Check sheet for the drawn part. Datum: minimum x, y, z corner. Units: mm. A direction names the side the tool comes from. Round coordinates to 2 decimals unless told otherwise and drop trailing zeros. Write each loop counter-clockwise with the first axis right and the second up, starting at its lowest first coordinate (ties: lowest second). Pieces come first, ordered by that corner, then holes.
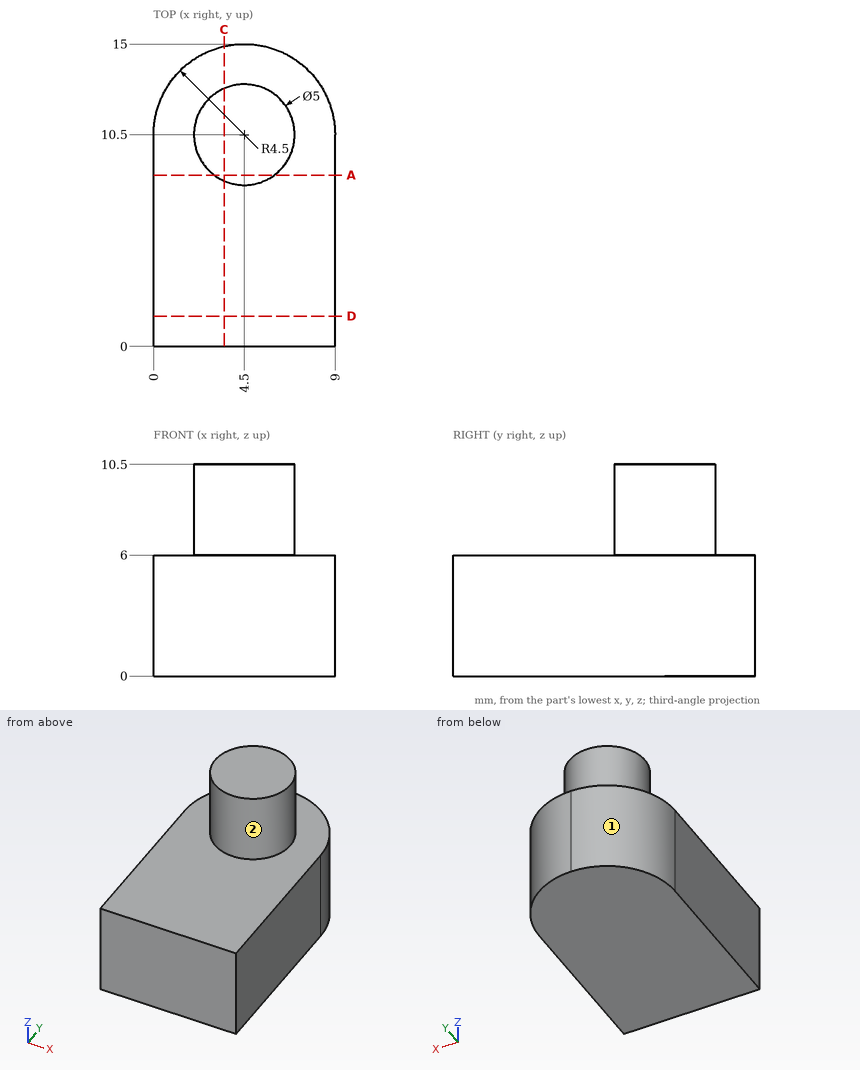
Q1. Tool access check on the marked faces 1 and 2. Record the directions out of +Z, -Z, +X, -X, +Y, -Y that give a thin tool (end or side, any length) a straight path to the whole face; none if there is none.
Recorded:
face 1: +Z, -Z, -X, +Y
face 2: +Z
Q2. Depth check by flat-ended pin: P1, Ø4, axis at x = 2.5, y = 4.5, coming from the -Z side; P2, Ø4, axis at y = 8.5, z = 9, coming from the -X side; P3, Ø1, axis at y = 6, z = 7, coming from the -X side; P4, Ø4, axis at x = 1.5, z = 3.5, coming from the +Y side. Enter the tip coordinate at first touch or a pass-through.
Recorded:
P1: stops at z = 0
P2: stops at x = 2
P3: passes through
P4: stops at y = 14.89
Q3. Material ranges on line 1 along Z through (x, y) = (2, 1.5); line 2 along Y through (x, z) = (4.75, 10); line 3 along X through (y, z) = (14, 4.25), recorded low to high.
Recorded:
line 1: z = 0 to 6
line 2: y = 8.01 to 12.99
line 3: x = 1.67 to 7.33
Q4. Sectioned sample at A-A (y = 8.5). Enter the section's corners in (x, z), plus the area to 3 significant figures.
Recorded:
outline: (0, 0) - (9, 0) - (9, 6) - (6, 6) - (6, 10.5) - (3, 10.5) - (3, 6) - (0, 6) - close
area: 67.5 mm2
Q5. Sectioned sample at C-C (x = 3.5). Enter the section's corners in (y, z), plus the area to 3 significant figures.
Recorded:
outline: (0, 0) - (14.89, 0) - (14.89, 6) - (12.79, 6) - (12.79, 10.5) - (8.21, 10.5) - (8.21, 6) - (0, 6) - close
area: 110 mm2
Q6. Sectioned sample at D-D (y = 1.5). Enter the section's corners in (x, z).
Recorded:
outline: (0, 0) - (9, 0) - (9, 6) - (0, 6) - close
